Build history of the part. All positions in model axes, mm. A direction names the side the tool comes from. Give positions to 0.01 mm unless a question says otherwise; leave off trailing zeros. Loops run counter-clockwise (first coordinate to the right, second up) from the corner with the lowest first, then second, coordinate; pieces in that order, holes last. Notation, with made-up numbers: (70.25, 44) - (126.25, 44) arc R29 cw to (126.25, 67) - close; hole circle Ø8 at (-29.75, 32.5). An arc over 180 degrees is marked (long way). Return JSON: item names as keys, results as strings. Group by question number.
1) Slice it at C-C (z = 1). List the corners of the cut face in (x, y), and give its area (3 significant figures).
2) Slice it at A-A (z = 12.5). List the corners of the cut face in (x, y).
3) Drill centre lines: probe 1 along X at (y, z) = (8.4, 12.5); probe 2 along Z at (x, y) = (60, 6.8); probe 3 along Y at (x, z) = (57, 26). Where is each one in solid material? Low to high. Write a range as from..to.
4) Slice it at D-D (x = 46). List the corners of the cut face in (y, z), and give its area (4 significant figures).
5) Slice it at B-B (x = 10). List the corners of the cut face in (y, z).
6) Drop flat-ended pins along their axis: pin 1 (3 mm diameter, centred on y = 28, z = 26, fed in from +X); pin 2 (12.5 mm diameter, centred on x = 40, z = 20.5, fed in from +Y); pin 3 (1.5 mm diameter, centred on x = 38.5, y = 48.5, fed in from +Z). Give the stop position or say it passes through.
7) Mould opens along Z. For faces 5 (the face through (35, 25, 0)), 6 (the face through (70, 44, 9)), 7 (the face through (14.77, 7.46, 11)), 8 (the face through (56.315, 7.465, 9.121)) say: released by +Z, released by -Z, zero draft, split by the parting line, or undercut.
8) 3-axis set-ups, long thin cutter, end or side, ignore diameter. For faces 1 (the face through (35, 2, 0)), 2 (the face through (14, 10, 16)), 3 (the face through (50, 25, 13)), 4 (the face through (35, 45, 17)): which of +Z, -Z, +X, -X, +Y, -Y reach the whole face in a straight line?
```python
from build123d import *

# Parameters (mm, degrees)
SKETCH1_W           = 70
SKETCH1_H           = 5
BOSS_EXTRUDE1_DEPTH = 10
SKETCH2_W           = 70
SKETCH2_H           = 5
BOSS_EXTRUDE2_DEPTH = 30
SKETCH3_R           = 5
CUT_EXTRUDE2_DEPTH  = 10
SKETCH4_R           = 5
CUT_EXTRUDE3_DEPTH  = 10
SKETCH6_W           = 30
SKETCH6_H           = 35
BOSS_EXTRUDE4_DEPTH = 30
BOSS_EXTRUDE5_DEPTH = 5
SKETCH8_W           = 70
SKETCH8_H           = 10
BOSS_EXTRUDE6_DEPTH = 5
SKETCH9_R           = 10
CUT_EXTRUDE4_DEPTH  = 30


with BuildPart() as part:
    # Sketch1 → Boss-Extrude1 (new body)
    with BuildSketch(Plane(origin=(0, 0, 0), x_dir=(1, 0, 0), z_dir=(0, 1, 0))):
        with Locations((35, 2.5)):
            Rectangle(SKETCH1_W, SKETCH1_H)
    extrude(amount=BOSS_EXTRUDE1_DEPTH)

    # Sketch2 → Boss-Extrude2 (add)
    with BuildSketch(Plane.XY):
        with Locations((35, 7.5)):
            Rectangle(SKETCH2_W, SKETCH2_H)
    extrude(amount=BOSS_EXTRUDE2_DEPTH)

    # Sketch3 → Cut-Extrude2 (cut)
    with BuildSketch(Plane(origin=(0, 0, 0), x_dir=(1, 0, 0), z_dir=(0, 1, 0))):
        with Locations((60, -12.5)):
            Circle(SKETCH3_R)
    extrude(amount=CUT_EXTRUDE2_DEPTH, mode=Mode.SUBTRACT)

    # Sketch4 → Cut-Extrude3 (cut)
    with BuildSketch(Plane(origin=(0, 0, 0), x_dir=(1, 0, 0), z_dir=(0, 1, 0))):
        with Locations((10, -12.5)):
            Circle(SKETCH4_R)
    extrude(amount=CUT_EXTRUDE3_DEPTH, mode=Mode.SUBTRACT)

    # Sketch6 → Boss-Extrude4 (add)
    with BuildSketch(Plane(origin=(0, 10, 0), x_dir=(1, 0, 0), z_dir=(0, 1, 0))):
        with Locations((35, -12.5)):
            Rectangle(SKETCH6_W, SKETCH6_H)
    extrude(amount=BOSS_EXTRUDE4_DEPTH)

    # Sketch7 → Boss-Extrude5 (add)
    with BuildSketch(Plane(origin=(0, 40, 0), x_dir=(1, 0, 0), z_dir=(0, 1, 0))):
        Polygon((20, 5), (0, 5), (0, -30), (70, -30), (70, 5), align=None)
    extrude(amount=BOSS_EXTRUDE5_DEPTH)

    # Sketch8 → Boss-Extrude6 (add)
    with BuildSketch(Plane(origin=(0, 45, 0), x_dir=(1, 0, 0), z_dir=(0, 1, 0))):
        with Locations((35, 0)):
            Rectangle(SKETCH8_W, SKETCH8_H)
    extrude(amount=BOSS_EXTRUDE6_DEPTH)

    # Sketch9 → Cut-Extrude4 (cut)
    with BuildSketch(Plane.XY.offset(30)):
        with Locations((35, 25)):
            Circle(SKETCH9_R)
    extrude(amount=-CUT_EXTRUDE4_DEPTH, mode=Mode.SUBTRACT)


solid = part.part
```
Results:
{
 "1": {"outline": "(0, 5) - (70, 5) - (70, 10) - (50, 10) - (50, 40) - (70, 40) - (70, 50) - (0, 50) - (0, 40) - (20, 40) - (20, 10) - (0, 10) - close; hole circle Ø20 at (35, 25)", "area": "1,640 mm2"},
 "2": {"outline": "(0, 5) - (5, 5) - (5, 10) - (0, 10) - close; (0, 40) - (20, 40) - (20, 10) - (15, 10) - (15, 5) - (55, 5) - (55, 10) - (50, 10) - (50, 40) - (70, 40) - (70, 45) - (0, 45) - close; (65, 5) - (70, 5) - (70, 10) - (65, 10) - close; hole circle Ø20 at (35, 25)"},
 "3": {"probe 1": "0..5, 15..55, 65..70", "probe 2": "-5..7.5, 17.5..30", "probe 3": "5..10, 40..45"},
 "4": {"outline": "(0, -5) - (50, -5) - (50, 5) - (45, 5) - (45, 30) - (5, 30) - (5, 0) - (0, 0) - close", "area": "1,475 mm2"},
 "5": {"outline": "(0, -5) - (10, -5) - (10, 7.5) - (5, 7.5) - (5, 0) - (0, 0) - close; (5, 17.5) - (10, 17.5) - (10, 30) - (5, 30) - close; (40, -5) - (50, -5) - (50, 5) - (45, 5) - (45, 30) - (40, 30) - close"},
 "6": {"pin 1": "x = 50", "pin 2": "y = 45", "pin 3": "z = 5"},
 "7": {"face 5": "released by +Z", "face 6": "zero draft", "face 7": "undercut", "face 8": "undercut"},
 "8": {"face 1": "+Z, +X, -X, -Y", "face 2": "+Z, -Z, -X", "face 3": "+Z, -Z, +X", "face 4": "+Z, +X, -X, +Y"}
}
